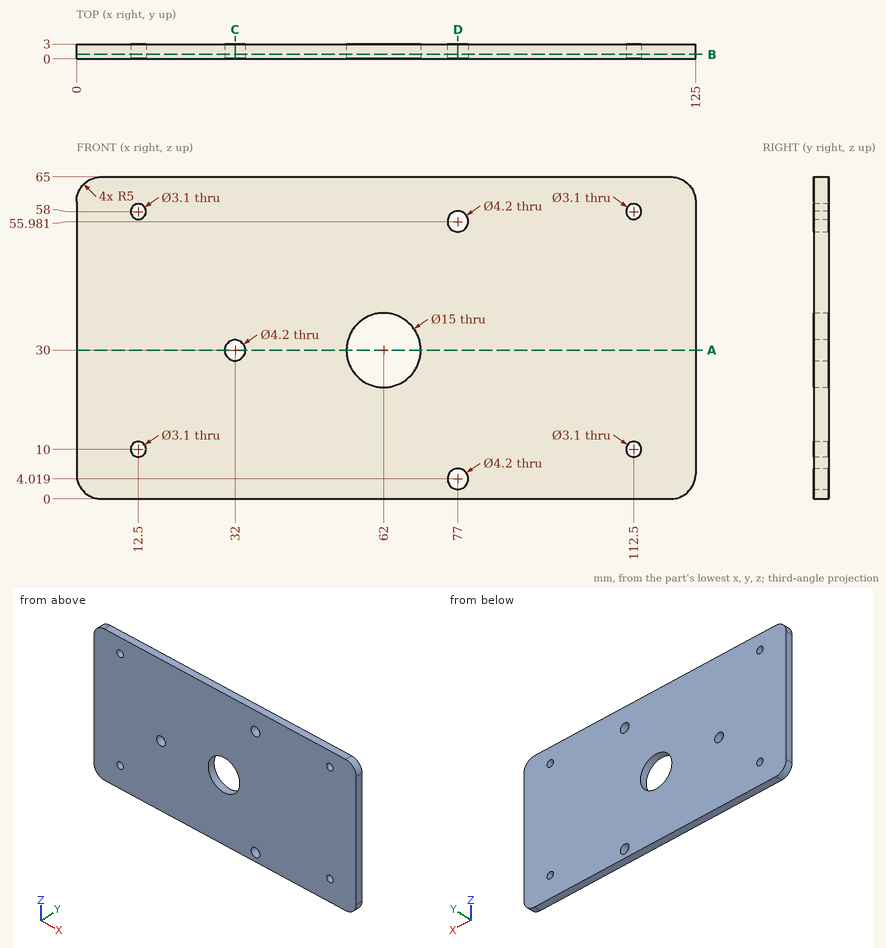
Source: three-view drawing plus pictorial views. Frame: mm from the lowest corner of the part. Coordinates: 2 decimals unless noted, no trailing zeros. Loops run counter-clockwise (first coordinate to the right, second up) from the corner with the lowest first, then second, coordinate; pieces in that order, holes last. Notation, with made-up numbers: M 30.25,-13 L 82.25,-13 A25 ccw 82.25,10 Z; hole C -29.75,-24 d9. An arc over 180 degrees is marked long. Use CSV: the item, a comma, the result in double quotes.
(1) Cut plane C-C on x = 32. Return loops of the section in (y, z).
Answers follow:
outline,"M 0,0 L 3,0 L 3,27.9 L 0,27.9 Z; M 0,32.1 L 3,32.1 L 3,65 L 0,65 Z"
(2) Cut plane A-A on z = 30. Return loops of the section in (x, y).
Answers follow:
outline,"M 0,0 L 29.9,0 L 29.9,3 L 0,3 Z; M 34.1,0 L 54.5,0 L 54.5,3 L 34.1,3 Z; M 69.5,0 L 125,0 L 125,3 L 69.5,3 Z"
(3) Line query: line 1 (X direction, y = 0.9, z = 10); line 2 (Z direction, x = 112.5, y = 2.05); line 3 (X direction, y = 1.45, z = 30). Output: solid intervals per line, ascending. Write a range as [from, to].
Answers follow:
line 1,"[0, 10.95], [14.05, 110.95], [114.05, 125]"
line 2,"[0, 8.45], [11.55, 56.45], [59.55, 65]"
line 3,"[0, 29.9], [34.1, 54.5], [69.5, 125]"
(4) Cut plane B-B on y = 0.9. Give the number of separate pieces and of enclosed holes in the cut face, and give its area (4 significant figures).
Answers follow:
separate pieces,"1"
enclosed holes,"8"
area,"7,855 mm²"
(5) Cut plane D-D on x = 77. Return loops of the section in (y, z).
Answers follow:
outline,"M 0,0 L 3,0 L 3,1.92 L 0,1.92 Z; M 0,6.12 L 3,6.12 L 3,53.88 L 0,53.88 Z; M 0,58.08 L 3,58.08 L 3,65 L 0,65 Z"
